Part model, mm, in its own coordinate system. A direction names the side the tool comes from. Round coordinates to 2 decimals unless told otherwise and drop trailing zeros. Write each loop counter-clockwise with the first axis right and the second up, starting at its lowest first coordinate (ties: lowest second). Pieces come first, ordered by that corner, then holes.
1) Pull direction X, two halves, no side cores. Call faces 1 (the flat face through (17, 2, 1)), 2 (the cylindrical face through (-15.928, 15.394, 0.493)): +X half, -X half, draft (parallel to the pull), parting line (faces both ways), or undercut.
2) Saw through at C-C on z = 0.4. Count the separate pieces of the cut face and the enclosed holes in it, and give its area (3 significant figures).
3) Saw through at A-A on y = 0.85. Write the cut outline in (x, z), and give its area (3 significant figures).
4) Drill centre lines: L1, parallel to X at y = 14, z = 0.2; L2, parallel to X at y = 2.5, z = 0.15; L3, parallel to X at y = 14.5, z = 0.55. Where is each one in solid material? Low to high.
5) Saw through at B-B on y = 6.5. Write the cut outline in (x, z).
6) Which spindle directions (+Z, -Z, +X, -X, +Y, -Y) get a long thin tool onto all of the face, cutting with end or side? Do faces 3 (the flat face through (17, 2, 0)), 4 (the flat face through (-2.089, 6.447, 0.493)). Say none if no direction does.
```python
from build123d import *

# Parameters (mm, degrees)
SKETCH1_W           = 80.536494558
SKETCH1_H           = 18.639450705
SKETCH1_R           = 1
SKETCH1_W_2         = 12.7
SKETCH1_H_2         = 10.505884886
SKETCH1_R_2         = 5.85
BOSS_EXTRUDE1_DEPTH = 1


with BuildPart() as part:
    # Sketch1 → Boss-Extrude1 (new body)
    with BuildSketch(Plane.XY):
        with Locations((8.176740168, 8.08881823)):
            Rectangle(SKETCH1_W, SKETCH1_H)
        with Locations((-23.606833594, 0.85)):
            Circle(SKETCH1_R, mode=Mode.SUBTRACT)
        with Locations((-14.928531322, 0.85)):
            Circle(SKETCH1_R, mode=Mode.SUBTRACT)
        with BuildLine():
            Line((-1.215095217, 5.746392688), (-2.98864341, 7.166966689))
            ThreePointArc((-2.98864341, 7.166966689), (-3.191938605, 7.422731407), (-3.264469824, 7.741296549))
            Line((-3.264469824, 7.741296549), (-3.264469824, 9.837116478))
            ThreePointArc((-3.264469824, 9.837116478), (-3.048943677, 10.357442625), (-2.52861753, 10.572968772))
            Line((-2.52861753, 10.572968772), (10.728001089, 10.572968772))
            ThreePointArc((10.728001089, 10.572968772), (11.248327236, 10.357442625), (11.463853383, 9.837116478))
            Line((11.463853383, 9.837116478), (11.463853383, 7.741296549))
            ThreePointArc((11.463853383, 7.741296549), (11.391322164, 7.422731407), (11.188026969, 7.166966689))
            Line((11.188026969, 7.166966689), (9.414478776, 5.746392688))
            ThreePointArc((9.414478776, 5.746392688), (9.198232155, 5.626424146), (8.954452897, 5.584870255))
            Line((8.954452897, 5.584870255), (-0.755069338, 5.584870255))
            ThreePointArc((-0.755069338, 5.584870255), (-0.998848596, 5.626424146), (-1.215095217, 5.746392688))
        make_face(mode=Mode.SUBTRACT)
        with Locations((22.024917985, 8.038348308)):
            Rectangle(SKETCH1_W_2, SKETCH1_H_2, mode=Mode.SUBTRACT)
        with Locations((41.175605906, 7.741296549)):
            Circle(SKETCH1_R_2, mode=Mode.SUBTRACT)
        with BuildLine():
            Line((-27.44598473, 14.1), (-27.44598473, 12.318789547))
            ThreePointArc((-27.44598473, 12.318789547), (-26.843437597, 11.871801459), (-26.613964343, 11.157516205))
            Line((-26.613964343, 11.157516205), (-26.613964343, 5.042483795))
            ThreePointArc((-26.613964343, 5.042483795), (-26.843437597, 4.328198541), (-27.44598473, 3.881210453))
            Line((-27.44598473, 3.881210453), (-27.44598473, 2.1))
            ThreePointArc((-27.44598473, 2.1), (-27.94598473, 1.6), (-28.44598473, 2.1))
            Line((-28.44598473, 2.1), (-28.44598473, 3.881210453))
            ThreePointArc((-28.44598473, 3.881210453), (-29.048531864, 4.328198541), (-29.278005117, 5.042483795))
            Line((-29.278005117, 5.042483795), (-29.278005117, 11.157516205))
            ThreePointArc((-29.278005117, 11.157516205), (-29.048531864, 11.871801459), (-28.44598473, 12.318789547))
            Line((-28.44598473, 12.318789547), (-28.44598473, 14.1))
            ThreePointArc((-28.44598473, 14.1), (-27.94598473, 14.6), (-27.44598473, 14.1))
        make_face(mode=Mode.SUBTRACT)
        with BuildLine():
            ThreePointArc((-17.992266615, 5.042483795), (-18.213073344, 4.340452327), (-18.79598473, 3.891210622))
            Line((-18.79598473, 3.891210622), (-18.79598473, 2.1))
            ThreePointArc((-18.79598473, 2.1), (-19.29598473, 1.6), (-19.79598473, 2.1))
            Line((-19.79598473, 2.1), (-19.79598473, 3.891210622))
            ThreePointArc((-19.79598473, 3.891210622), (-20.378896116, 4.340452327), (-20.599702845, 5.042483795))
            Line((-20.599702845, 5.042483795), (-20.599702845, 11.157516205))
            ThreePointArc((-20.599702845, 11.157516205), (-20.378896116, 11.859547673), (-19.79598473, 12.308789378))
            Line((-19.79598473, 12.308789378), (-19.79598473, 14.1))
            ThreePointArc((-19.79598473, 14.1), (-19.29598473, 14.6), (-18.79598473, 14.1))
            Line((-18.79598473, 14.1), (-18.79598473, 12.308789378))
            ThreePointArc((-18.79598473, 12.308789378), (-18.213073344, 11.859547673), (-17.992266615, 11.157516205))
            Line((-17.992266615, 11.157516205), (-17.992266615, 5.042483795))
        make_face(mode=Mode.SUBTRACT)
        with BuildLine():
            Line((-10.14598473, 14.1), (-10.14598473, 12.318789547))
            ThreePointArc((-10.14598473, 12.318789547), (-9.543437597, 11.871801459), (-9.313964343, 11.157516205))
            Line((-9.313964343, 11.157516205), (-9.313964343, 5.042483795))
            ThreePointArc((-9.313964343, 5.042483795), (-9.543437597, 4.328198541), (-10.14598473, 3.881210453))
            Line((-10.14598473, 3.881210453), (-10.14598473, 2.1))
            ThreePointArc((-10.14598473, 2.1), (-10.64598473, 1.6), (-11.14598473, 2.1))
            Line((-11.14598473, 2.1), (-11.14598473, 3.881210453))
            ThreePointArc((-11.14598473, 3.881210453), (-11.748531864, 4.328198541), (-11.978005117, 5.042483795))
            Line((-11.978005117, 5.042483795), (-11.978005117, 11.157516205))
            ThreePointArc((-11.978005117, 11.157516205), (-11.748531864, 11.871801459), (-11.14598473, 12.318789547))
            Line((-11.14598473, 12.318789547), (-11.14598473, 14.1))
            ThreePointArc((-11.14598473, 14.1), (-10.64598473, 14.6), (-10.14598473, 14.1))
        make_face(mode=Mode.SUBTRACT)
        with Locations((-23.606833594, 15.35)):
            Circle(SKETCH1_R, mode=Mode.SUBTRACT)
        with Locations((-14.928531322, 15.35)):
            Circle(SKETCH1_R, mode=Mode.SUBTRACT)
        with Locations((22.024917985, 15.541290751)):
            Circle(SKETCH1_R, mode=Mode.SUBTRACT)
    extrude(amount=BOSS_EXTRUDE1_DEPTH)


solid = part.part
```
Completed:
1. face 1: draft
1. face 2: undercut
2. separate pieces: 1
2. enclosed holes: 11
2. area: 1,100 mm2
3. outline: (-32.09, 0) - (-24.61, 0) - (-24.61, 1) - (-32.09, 1) - close; (-22.61, 0) - (-15.93, 0) - (-15.93, 1) - (-22.61, 1) - close; (-13.93, 0) - (48.44, 0) - (48.44, 1) - (-13.93, 1) - close
3. area: 76.5 mm2
4. L1: x = -32.09 to -28.45, -27.45 to -19.8, -18.8 to -11.15, -10.15 to 48.44
4. L2: x = -32.09 to -28.45, -27.45 to -19.8, -18.8 to -11.15, -10.15 to 38.58, 43.77 to 48.44
4. L3: x = -32.09 to -28.25, -27.65 to -24.13, -23.08 to -19.6, -19 to -15.46, -14.4 to -10.95, -10.35 to 48.44
5. outline: (-32.09, 0) - (-29.28, 0) - (-29.28, 1) - (-32.09, 1) - close; (-26.61, 0) - (-20.6, 0) - (-20.6, 1) - (-26.61, 1) - close; (-17.99, 0) - (-11.98, 0) - (-11.98, 1) - (-17.99, 1) - close; (-9.31, 0) - (-2.16, 0) - (-2.16, 1) - (-9.31, 1) - close; (10.36, 0) - (15.67, 0) - (15.67, 1) - (10.36, 1) - close; (28.37, 0) - (35.46, 0) - (35.46, 1) - (28.37, 1) - close; (46.89, 0) - (48.44, 0) - (48.44, 1) - (46.89, 1) - close
6. face 3: -Z, +X, -X, +Y, -Y
6. face 4: +Z, -Z
